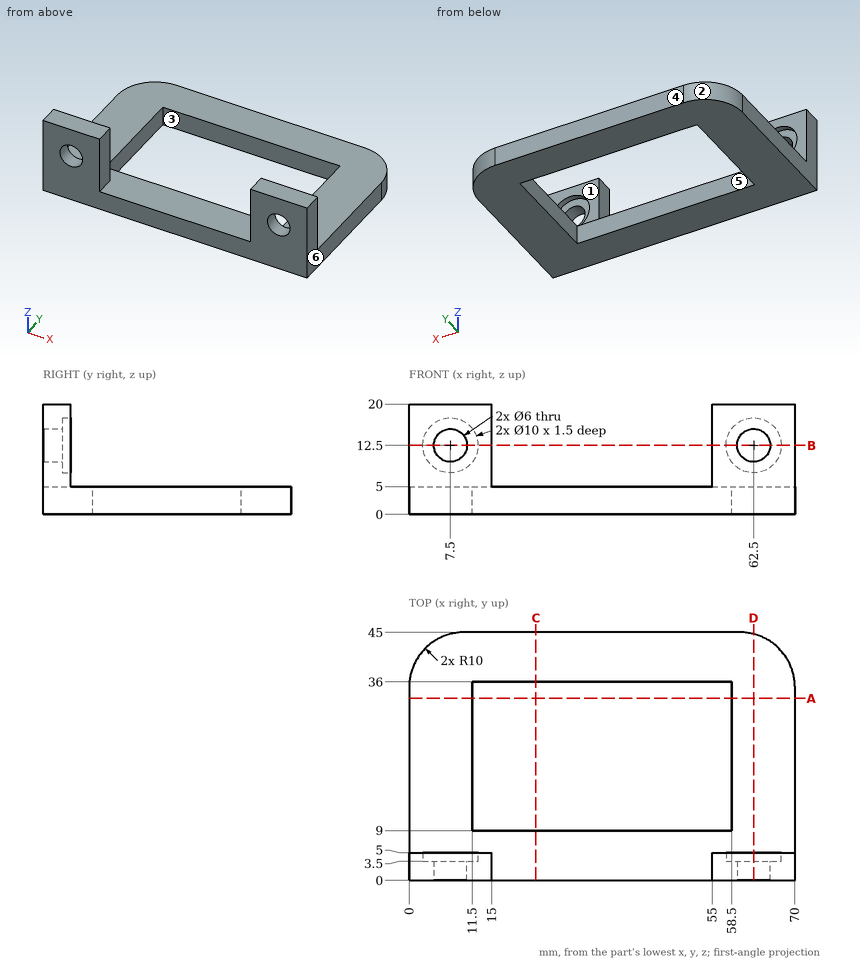
Can you work these out from the drawing? Everything is in mm from the part's minimum corner. A direction names the side the tool comes from. Give positions to 0.01 mm unless a question says otherwise; leave off trailing zeros. Order: outer loops, then holes, each group sorted by start corner. A loop starts at its lowest first (then second) coordinate and runs counter-clockwise, first axis right, second up. Notation, with made-up numbers: M 44,60 L 101,60 A8 cw 101,67 Z; hole C 38.5,-7.75 d8. An arc over 180 degrees is marked long. Write item = value, one per line. Start each with the question number.
Q1. Suppose I cut it at A-A (y = 33). Write out the boundary of the cut face in (x, z).
Q2. I need wall thicknesses on probe 1 along Z at (x, y) = (62.5, 4.6); probe 2 along X at (y, z) = (10, 3.75); probe 3 along Y at (x, z) = (21, 1). Which ranges of each line are inside material? Lowest first, please. Write a range as [from, to].
Q3. For the marked faces 1, 2 and 3, which set-ups out of +Z, -Z, +X, -X, +Y, -Y let a thin tool reach every point of the face, with its end or its side?
Q4. We'd pull the mould along X, two halves only. Please class the marked faces 4, 5 and 6: pulls with the +X half, pulls with the -X half, needs draft (parallel to the pull), parting line crosses it, or undercut.
Q5. Suppose I cut it at C-C (x = 23). Write out the boundary of the cut face in (y, z).
Q6. Suppose I cut it at D-D (x = 62.5). Write out the boundary of the cut face in (y, z), plus the area to 3 significant figures.
Q7. Suppose I cut it at B-B (z = 12.5). Write out the boundary of the cut face in (x, y), plus the area to 3 significant figures.
Q8. Will these pins go through, and if not, where does the flat tip stop? pin 1 Ø7.5 at (x, z) = (10, 13.5) entering from +Y; pin 2 Ø9 at (x, z) = (7.5, 12.5) entering from +Y; pin 3 Ø5 at (x, z) = (7.5, 12.5) entering from +Y; pin 4 Ø4 at (x, z) = (62.5, 3) entering from -Y.
Check result:
q1.outline = M 0,0 L 11.5,0 L 11.5,5 L 0,5 Z; M 58.5,0 L 70,0 L 70,5 L 58.5,5 Z
q2.probe_1 = [0, 7.5], [17.5, 20]
q2.probe_2 = [0, 11.5], [58.5, 70]
q2.probe_3 = [0, 9], [36, 45]
q3.face_1 = +Z, +X, -X, +Y
q3.face_2 = +Z, -Z, -X, +Y
q3.face_3 = +Z, -Z
q4.face_4 = needs draft
q4.face_5 = undercut
q4.face_6 = pulls with the +X half
q5.outline = M 0,0 L 9,0 L 9,5 L 0,5 Z; M 36,0 L 45,0 L 45,5 L 36,5 Z
q6.outline = M 0,0 L 44.68,0 L 44.68,5 L 5,5 L 5,7.5 L 3.5,7.5 L 3.5,9.5 L 0,9.5 Z; M 0,15.5 L 3.5,15.5 L 3.5,17.5 L 5,17.5 L 5,20 L 0,20 Z
q6.area = 262 mm2
q7.outline = M 0,0 L 4.5,0 L 4.5,3.5 L 2.5,3.5 L 2.5,5 L 0,5 Z; M 10.5,0 L 15,0 L 15,5 L 12.5,5 L 12.5,3.5 L 10.5,3.5 Z; M 55,0 L 59.5,0 L 59.5,3.5 L 57.5,3.5 L 57.5,5 L 55,5 Z; M 65.5,0 L 70,0 L 70,5 L 67.5,5 L 67.5,3.5 L 65.5,3.5 Z
q7.area = 78.0 mm2
q8.pin_1 = 5
q8.pin_2 = 3.5
q8.pin_3 = through
q8.pin_4 = 0
